```python
from build123d import *

# Parameters (mm, degrees)
F1_DEPTH    = 38.1
F2_T1_DEPTH = 161.0672212421
F4_D        = 9.525
F5_R        = 1
F6_DEPTH    = 6.35


# Not quite as in the source:
# - a fillet or chamfer that OpenCascade refuses, or shapes differently, is made with other operations: its cross-section is extruded or revolved along the edge and cut away or added


with BuildPart() as f1:
    # F0 (on Front) → F1 (new body)
    with BuildSketch(Plane.XZ):
        with BuildLine():
            Line((37.3479522824, 5.9316984817), (-32.5020477176, 5.9316984817))
            Line((-32.5020477176, 5.9316984817), (-32.5020477176, -13.1183015183))
            Line((-32.5020477176, -13.1183015183), (37.3479522824, -13.1183015183))
            ThreePointArc((37.3479522824, -13.1183015183), (46.8729522824, -3.5933015183), (37.3479522824, 5.9316984817))
        make_face()
    extrude(amount=F1_DEPTH)

    # F2: fillet of radius 25.4 on 1 edges, made by hand

    # F2_s2 → F2_t1 (cut)
    with BuildSketch(Plane.XZ.offset(-61.483610621)):
        with BuildLine():
            ThreePointArc((-32.5020477176, 5.9316984817), (-23.4628633358, -7.7987646603), (-7.9086034692, -13.1183015183))
            Line((-7.9086034692, -13.1183015183), (-32.5020477176, -13.1183015183))
            Line((-32.5020477176, -13.1183015183), (-32.5020477176, 5.9316984817))
        make_face()
    extrude(amount=F2_T1_DEPTH, mode=Mode.SUBTRACT)

    # F4 (through all)
    with Locations(Plane.XZ.offset(38.1)):
        with Locations((37.3479522824, -3.5933015183)):
            Hole(F4_D / 2)

    # F5 (on face) → F6 (join)
    with BuildSketch(Plane.XY.offset(5.9316984817)):
        with Locations((-24.94562231, -19.05)):
            Circle(F5_R)
    extrude(amount=F6_DEPTH)


solid = f1.part
```
Can you work these out from the model? Positions are in its coordinate system, mm. Give positions to 0.01 mm unless a question says otherwise; leave off trailing zeros. Loops run counter-clockwise (first coordinate to the right, second up) from the corner with the lowest first, then second, coordinate; pieces in that order, holes last. Notation, with made-up numbers: M 74,-14 L 78,-14 A16 cw 78,2 Z; hole C 60.25,-13.75 d4. An arc over 180 degrees is marked long. Use CSV: the item, a comma, the result in double quotes. Start each with the question number.
1. Imagine slicing it at D-D, the plane x = -0.5. Write out the boundary of the cut face in (y, z).
2. If I drill on L1, parallel to Z at x = 8.5, y = -14; L2, parallel to X at y = -7, z = -1.75; L3, parallel to Z at x = 40, y = -24.5, over which ranges is the centre line in solid material (lowest first)?
3. Imagine slicing it at C-C, the plane z = 7.25. Write out the boundary of the cut face in (x, y), plus the area to 3 significant figures.
4. Imagine slicing it at A-A, the plane z = -5.25. Write out the boundary of the cut face in (x, y).
5. For P1, Ø5, axis at x = 30, y = -31.5, coming from the +Z side; P2, Ø12, axis at y = -19.5, z = -4.5, coming from the +X side; P3, Ø8, axis at y = -7, z = 8.5, coming from the +X side, each with a flat end and sliding along its axis, tell me the tip position at first contact or that it passes through.
6. If we mould it in two halves opening along X, with no side actions, what happens to faces 1 (the face through (-25, -19, 12.282)), 2 (the face through (42.106, -18.783, -3.384)), 3 (the face through (-25.74, -19.66, 9.06)), 4 (the face through (46.87, -18.78, -3.8))? For each: released by +X, released by -X, zero draft, split by the parting line, or undercut.
Response values:
1,outline,"M -38.1,-13.12 L 0,-13.12 L 0,5.93 L -38.1,5.93 Z"
2,L1,"-13.12 to 5.93"
2,L2,"-29.08 to 32.96, 41.74 to 46.69"
2,L3,"-12.74 to -7.55, 0.36 to 5.56"
3,outline,"C -24.95,-19.05 d2"
3,area,"3.14 mm^2"
4,outline,"M -26.29,-38.1 L 32.88,-38.1 L 32.88,0 L -26.29,0 Z; M 41.81,-38.1 L 46.73,-38.1 L 46.73,0 L 41.81,0 Z"
5,P1,"z = 5.93"
5,P2,"x = 46.87"
5,P3,"x = 42.37"
6,face 1,"zero draft"
6,face 2,"undercut"
6,face 3,"split by the parting line"
6,face 4,"released by +X"
